CAD build for the part. Positions are in the model's coordinates, mm. A direction names the side the tool comes from. Coordinates: 2 decimals unless noted, no trailing zeros. Loops run counter-clockwise (first coordinate to the right, second up) from the corner with the lowest first, then second, coordinate; pieces in that order, holes last.
1) Which spindle directions (+Z, -Z, +X, -X, +Y, -Y) get a long thin tool onto all of the face, cutting with end or side? Do faces 4 (the flat face through (34, 15, -25)), 5 (the flat face through (0, 7, -14)), 6 (the flat face through (66.04, 7, 1)), 7 (the flat face through (66.04, 7, -45)). Say none if no direction does.
2) Wall check: line 1 along X through (y, z) = (9, -48.26); line 2 along X through (y, z) = (11.75, -5.08); line 3 along X through (y, z) = (8, -27). Give the ranges that are in metal, low to high.
3) Two-plate mould, pull along Z, no slides. Class faces 1 (the cylindrical face through (67.39, 7.4, -4.22)), 2 (the flat face through (0, 7, -45)), 3 (the flat face through (33, 7, 2.54)): +Z half, -Z half, draft (parallel to the pull), parting line (faces both ways), or undercut.
4) Saw through at D-D, the plane z = -5.08. Write the cut outline in (x, y).
5) Pin check, flat tip, straight feed: pin 1 Ø2 at (y, z) = (3, -41.5) entering from -X. Stop position of the tip, or through.
6) Saw through at B-B, the plane x = 15.24. Write the cut outline in (y, z), and give its area (3 significant figures).
7) Saw through at A-A, the plane z = -48.26. Write the cut outline in (x, y), and give its area (3 significant figures).
8) Saw through at C-C, the plane y = 5.25. Write the cut outline in (x, z).
```python
from build123d import *

# Parameters (mm, degrees)
SZKIC1_R                    = 1.6
DODANIE_WYCI_GNI_CIE1_DEPTH = 15
SZKIC2_W                    = 2
SZKIC2_H                    = 9
WYTNIJ_WYCI_GNI_CIE1_DEPTH  = 88.018168218


with BuildPart() as part:
    # Szkic1 → Dodanie-wyciągnięcie1 (new body)
    with BuildSketch(Plane(origin=(0, 0, 0), x_dir=(1, 0, 0), z_dir=(0, 1, 0))):
        Polygon((0, -2.54), (66.04, -2.54), (66.04, 0), (69.04, 3), (69.04, 36.5), (66.04, 39.5), (66.04, 50.8), (0, 50.8), (0, 38.8), (-1, 38.8), (-1, 30.8), (0, 30.8), (0, 9), (-2, 9), (-2, 0), (0, 0), align=None)
        with Locations(Location((15.24, 0, 0), (0, 0, 270))):
            Circle(SZKIC1_R, mode=Mode.SUBTRACT)
        with Locations(Location((66.04, 33.02, 0), (0, 0, 270))):
            Circle(SZKIC1_R, mode=Mode.SUBTRACT)
        with Locations(Location((66.04, 5.08, 0), (0, 0, 270))):
            Circle(SZKIC1_R, mode=Mode.SUBTRACT)
        with Locations(Location((15.24, 48.26, 0), (0, 0, 270))):
            Circle(SZKIC1_R, mode=Mode.SUBTRACT)
    extrude(amount=DODANIE_WYCI_GNI_CIE1_DEPTH)

    # Szkic2 → Wytnij-wyciągnięcie1 (cut, through all)
    with BuildSketch(Plane(origin=(0, 15, 0), x_dir=(1, 0, 0), z_dir=(0, 1, 0))):
        with Locations((-1, 4.5)):
            Rectangle(SZKIC2_W, SZKIC2_H)
    extrude(amount=-WYTNIJ_WYCI_GNI_CIE1_DEPTH, mode=Mode.SUBTRACT)


solid = part.part
```
Data:
1. face 4: +Z, -Z, +X, -X, +Y
1. face 5: +Z, -X, +Y, -Y
1. face 6: +Z, +X, +Y, -Y
1. face 7: -Z, +X, +Y, -Y
2. line 1: x = 0 to 13.64, 16.84 to 66.04
2. line 2: x = 0 to 64.44, 67.64 to 69.04
2. line 3: x = 0 to 69.04
3. face 1: undercut
3. face 2: draft
3. face 3: +Z half
4. outline: (0, 0) - (64.44, 0) - (64.44, 15) - (0, 15) - close; (67.64, 0) - (69.04, 0) - (69.04, 15) - (67.64, 15) - close
5. pin 1: stops at x = 0
6. outline: (0, -50.8) - (15, -50.8) - (15, -49.86) - (0, -49.86) - close; (0, -46.66) - (15, -46.66) - (15, -1.6) - (0, -1.6) - close; (0, 1.6) - (15, 1.6) - (15, 2.54) - (0, 2.54) - close
6. area: 704 mm2
7. outline: (0, 0) - (13.64, 0) - (13.64, 15) - (0, 15) - close; (16.84, 0) - (66.04, 0) - (66.04, 15) - (16.84, 15) - close
7. area: 943 mm2
8. outline: (-1, -38.8) - (0, -38.8) - (0, -50.8) - (66.04, -50.8) - (66.04, -39.5) - (69.04, -36.5) - (69.04, -3) - (66.04, 0) - (66.04, 2.54) - (0, 2.54) - (0, -30.8) - (-1, -30.8) - close; hole circle Ø3.2 at (15.24, -48.26); hole circle Ø3.2 at (15.24, 0); hole circle Ø3.2 at (66.04, -33.02); hole circle Ø3.2 at (66.04, -5.08)
